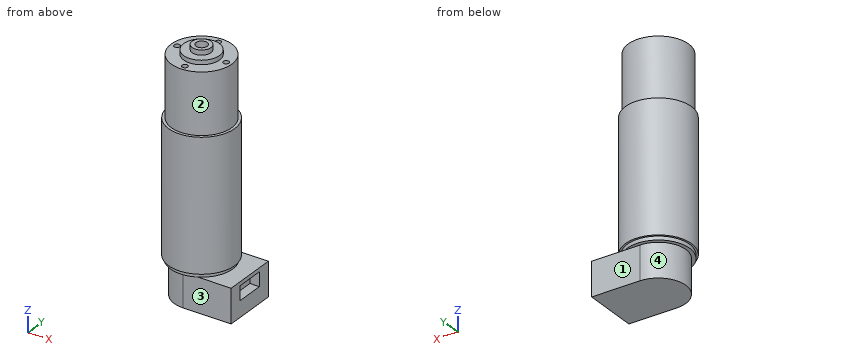
```python
from build123d import *

# Parameters (mm, degrees)
SKETCH_1_R               = 17.5
EXTRUDE_1_DEPTH          = 69
SKETCH_2_R               = 16
EXTRUDE_2_DEPTH          = 26
SKETCH_3_R               = 16
EXTRUDE_3_DEPTH          = 6
SKETCH_4_R               = 9.5
EXTRUDE_4_DEPTH          = 2.25
SKETCH_5_R               = 5
EXTRUDE_5_DEPTH          = 2.6
SKETCH_8_R               = 16.5
EXTRUDE_7_DEPTH          = 2
EXTRUDE_8_DEPTH          = 18
SKETCH_10_W              = 7.5
SKETCH_10_H              = 15
CUT_EXTRUDE_2_DEPTH      = 5
SKETCH_7_R               = 1.5
CUT_EXTRUDE_1_DEPTH      = 3.8
PATTERN_CIRCULAR_1_COUNT = 4
SKETCH_6_R               = 3
CUT_EXTRUDE_3_DEPTH      = 10


with BuildPart() as part:
    # 스케치1 → 보스-돌출1 (new body)
    with BuildSketch(Plane.XY):
        Circle(SKETCH_1_R)
    extrude(amount=EXTRUDE_1_DEPTH)

    # 스케치2 → 보스-돌출2 (add)
    with BuildSketch(Plane.XY.offset(69)):
        with Locations(Location((0, 0, 0), (0, 0, 180))):
            Circle(SKETCH_2_R)
    extrude(amount=EXTRUDE_2_DEPTH)

    # 스케치3 → 보스-돌출3 (add)
    with BuildSketch(Plane.XY.offset(95)):
        with Locations(Location((0, 0, 0), (0, 0, 180))):
            Circle(SKETCH_3_R)
    extrude(amount=EXTRUDE_3_DEPTH)

    # 스케치4 → 보스-돌출4 (add)
    with BuildSketch(Plane.XY.offset(101)):
        Circle(SKETCH_4_R)
    extrude(amount=EXTRUDE_4_DEPTH)

    # 스케치5 → 보스-돌출5 (add)
    with BuildSketch(Plane.XY.offset(103.25)):
        Circle(SKETCH_5_R)
    extrude(amount=EXTRUDE_5_DEPTH)

    # 스케치8 → 보스-돌출7 (add)
    with BuildSketch(Plane(origin=(0, 0, 0), x_dir=(-1, 0, 0), z_dir=(0, 0, -1))):
        with Locations(Location((0, 0, 0), (0, 0, 180))):
            Circle(SKETCH_8_R)
    extrude(amount=EXTRUDE_7_DEPTH)

    # 스케치9 → 보스-돌출8 (add)
    with BuildSketch(Plane(origin=(0, 0, -2), x_dir=(-1, 0, 0), z_dir=(0, 0, -1))):
        with BuildLine():
            Line((0, 14.5), (-25.5, 14.5))
            Line((-25.5, 14.5), (-25.5, -14.5))
            Line((-25.5, -14.5), (0, -14.5))
            ThreePointArc((0, -14.5), (14.5, 0), (0, 14.5))
        make_face()
    extrude(amount=EXTRUDE_8_DEPTH)

    # 스케치10 → 컷-돌출2 (cut)
    with BuildSketch(Plane(origin=(25.5, 0, 0), x_dir=(0, 0, -1), z_dir=(1, 0, 0))):
        with Locations((7.760897897, 0)):
            Rectangle(SKETCH_10_W, SKETCH_10_H)
    extrude(amount=-CUT_EXTRUDE_2_DEPTH, mode=Mode.SUBTRACT)

    # 스케치7 → 컷-돌출1 (cut)
    with BuildSketch(Plane.XY.offset(101)):
        with Locations((0, 13)):
            Circle(SKETCH_7_R)
    cut_extrude_1 = extrude(amount=-CUT_EXTRUDE_1_DEPTH, mode=Mode.SUBTRACT)

    # 원형 패턴1: 컷-돌출1 ×4 about axis
    pattern_circular_1_axis = Axis((0, 0, 0), (0, 0, 1))
    for i in range(1, PATTERN_CIRCULAR_1_COUNT):
        add(cut_extrude_1.rotate(pattern_circular_1_axis, i * 360 / PATTERN_CIRCULAR_1_COUNT), mode=Mode.SUBTRACT)

    # 스케치6 → 컷-돌출3 (cut)
    with BuildSketch(Plane.XY.offset(105.85)):
        Circle(SKETCH_6_R)
    extrude(amount=-CUT_EXTRUDE_3_DEPTH, mode=Mode.SUBTRACT)


solid = part.part
```
Source: CAD feature listing. Evaluate the final solid. Frame: model axes, mm. Face numbers are marked on the shaded views. A direction names the side the tool comes from. Round coordinates to 2 decimals unless told otherwise and drop trailing zeros. Loops run counter-clockwise (first coordinate to the right, second up) from the corner with the lowest first, then second, coordinate; pieces in that order, holes last. Notation, with made-up numbers: M 84,-29.5 L 128,-29.5 A21 cw 128,-21.5 Z; hole C 74,-12 d10. An arc over 180 degrees is marked long. Put each result on its own line as item: value.
(1) Ray query, line 1 (Z direction, x = 12.5, y = -12); line 2 (Z direction, x = 21.5, y = -5); line 3 (Z direction, x = 17, y = 10). Return the intervals inside material, ascending. Write a range as [from, to].
Solutions:
line 1: [-20, -2], [0, 69]
line 2: [-20, -11.51], [-4.01, -2]
line 3: [-20, -2]
(2) Section B-B, the plane z = 8. Return loops of the section in (x, y), and give its area (3 significant figures).
Solutions:
outline: C 0,0 d35
area: 962 mm²
(3) Section D-D, the plane z = 78. Return loops of the section in (x, y), and give its area (3 significant figures).
Solutions:
outline: C 0,0 d32
area: 804 mm²
(4) Section A-A, the plane x = 13. Return loops of the section in (y, z).
Solutions:
outline: M -14.5,-20 L 14.5,-20 L 14.5,-2 L 10.16,-2 L 10.16,0 L 11.72,0 L 11.72,69 L 9.33,69 L 9.33,101 L 1.5,101 L 1.5,97.2 L -1.5,97.2 L -1.5,101 L -9.33,101 L -9.33,69 L -11.72,69 L -11.72,0 L -10.16,0 L -10.16,-2 L -14.5,-2 Z
(5) Section C-C, the plane y = -13. Return loops of the section in (x, z), and give its area (3 significant figures).
Solutions:
outline: M -11.72,0 L -10.16,0 L -10.16,-2 L -6.42,-2 L -6.42,-20 L 25.5,-20 L 25.5,-2 L 10.16,-2 L 10.16,0 L 11.72,0 L 11.72,69 L 9.33,69 L 9.33,101 L 1.5,101 L 1.5,97.2 L -1.5,97.2 L -1.5,101 L -9.33,101 L -9.33,69 L -11.72,69 Z
area: 2,820 mm²
(6) Access query for the marked faces 1, 2, 3 and 4. Directions: +Z, -Z, +X, -X, +Y, -Y. A direction counts if a zero-diameter tool reaches every point of the face in a straight line with its end or side. Return the directions, or none.
Solutions:
face 1: -Z, +X, -X, +Y
face 2: +Z
face 3: -Z, +X, -X, -Y
face 4: -Z, -X
(7) First-contact query: pin 1 (4 mm diameter, centred on x = 24, y = -3.5, fed in from +Z); pin 2 (14.5 mm diameter, centred on x = 18, z = -8.5, fed in from +Y); pin 3 (5 mm diameter, centred on y = -1.5, z = 76, fed in from -X). Flat tips, straight axial feed; report the tip coordinate or a pass-through.
Solutions:
pin 1: z = -2
pin 2: y = 14.5
pin 3: x = -16
